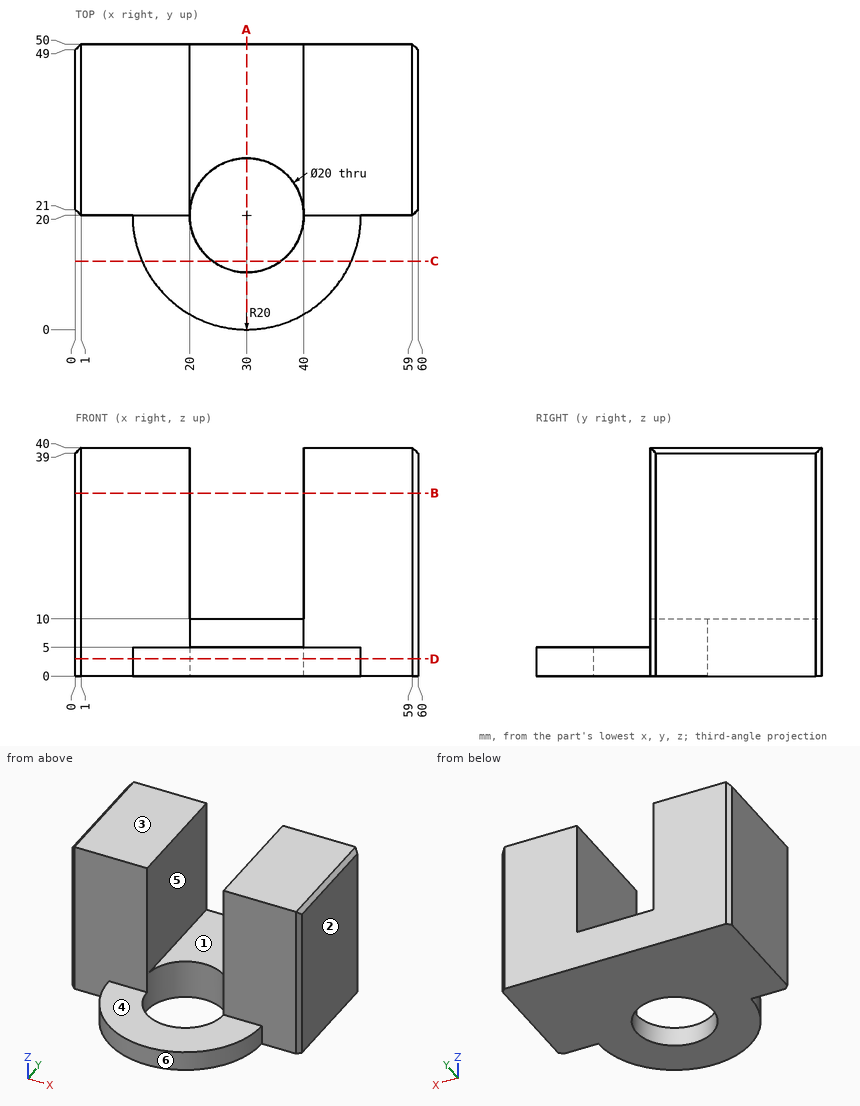
Study the drawing (mm; zero at the part's minimum x, y, z) and answer. A direction names the side the tool comes from. Give positions to 0.01 mm unless a question says otherwise; leave off trailing zeros. Write each loop counter-clockwise with the first axis right and the second up, starting at its lowest first coordinate (ties: lowest second). Pieces come first, ordered by that corner, then holes.
Item 1: Section C-C, the plane y = 12 is taken. Write down the section's boundary in (x, z), plus the area to 3 significant figures.
Item 2: Section B-B, the plane z = 32 is taken. Write down the section's boundary in (x, y), plus the area to 3 significant figures.
Item 3: Section D-D, the plane z = 3 is taken. Write down the section's boundary in (x, y), plus the area to 3 significant figures.
Item 4: Find the intervals of material crossed by line 1 along X through (y, z) = (34, 36); line 2 along Y through (x, z) = (5, 31); line 3 along Y through (x, z) = (30, 2), in increasing order.
Item 5: Determine the mould class of the marked faces 1, 2 and 3 for opening direction X: released by +X, released by -X, zero draft, split by the parting line, or undercut.
Item 6: Flat-ended cylindrical pins translate along their axes: P1, Ø9.5, axis at x = 8.5, z = 16.5, coming from the -Y side; P2, Ø8, axis at x = 35, y = 32, coming from the +Z side; P3, Ø10, axis at x = 32, y = 10, coming from the +Z side. Find the tip coordinate at first contact, or state that the pin passes through.
Item 7: Section A-A, the plane x = 30 is taken. Write down the section's boundary in (y, z), plus the area to 3 significant figures.
Item 8: Which of the six approach directions +Z, -Z, +X, -X, +Y, -Y give full straight-line access (tool end or side, diameter ignored) to the marked faces 4, 5 and 6?
Completed:
1. outline: (11.67, 0) - (24, 0) - (24, 5) - (11.67, 5) - close; (36, 0) - (48.33, 0) - (48.33, 5) - (36, 5) - close
1. area: 123 mm2
2. outline: (0, 21) - (1, 20) - (20, 20) - (20, 50) - (1, 50) - (0, 49) - close; (40, 20) - (59, 20) - (60, 21) - (60, 49) - (59, 50) - (40, 50) - close
2. area: 1,200 mm2
3. outline: (0, 21) - (1, 20) - (10, 20) arc R20 ccw to (50, 20) - (59, 20) - (60, 21) - (60, 49) - (59, 50) - (1, 50) - (0, 49) - close; hole circle Ø20 at (30, 20)
3. area: 2,110 mm2
4. line 1: x = 0 to 20, 40 to 60
4. line 2: y = 20 to 50
4. line 3: y = 0 to 10, 30 to 50
5. face 1: undercut
5. face 2: released by +X
5. face 3: zero draft
6. P1: stops at y = 20
6. P2: stops at z = 10
6. P3: stops at z = 5
7. outline: (0, 0) - (10, 0) - (10, 5) - (0, 5) - close; (30, 0) - (50, 0) - (50, 10) - (30, 10) - close
7. area: 250 mm2
8. face 4: +Z, +X, -X, -Y
8. face 5: +Z, +Y, -Y
8. face 6: +Z, -Z, -Y
